The listing builds one solid part. Answer for the finished solid, in the listing's coordinates (mm). Face numbers are marked on the shaded views. Round coordinates to 2 decimals unless told otherwise and drop trailing zeros. Write each loop counter-clockwise with the first axis right and the second up, starting at its lowest first coordinate (ties: lowest second). Pieces come first, ordered by that corner, then holes. Notation, with made-up numbers: (25, -36.75) - (84, -36.75) arc R18 ccw to (84, -17.75) - close; hole circle Ø1 at (-25.5, -13.5). An arc over 180 degrees is marked (long way). Answer as CSV lines item,"result". Start each with the question number.
Item 1: A cutting plane is placed at D-D on x = -5.25. Determine the outline of the cut face in (y, z).
Item 2: A cutting plane is placed at A-A on z = 2.5. Determine the outline of the cut face in (x, y), and give its area (3 significant figures).
Item 3: Flat-ended cylindrical pins translate along their axes: pin 1 (1 mm diameter, centred on x = 4, y = 1, fed in from -Z); pin 2 (1.8 mm diameter, centred on x = -8, z = -2.5, fed in from +Y); pin 3 (0.6 mm diameter, centred on x = 8.5, y = 1.5, fed in from -Z); pin 4 (1 mm diameter, centred on y = 1, z = 0, fed in from +X). Find the tip coordinate at first contact, or state that the pin passes through.
Item 4: For a pull along X with two mould halves and no side action, classify the marked faces 1 and 2 as pulls with the +X half, pulls with the -X half, needs draft (parallel to the pull), parting line crosses it, or undercut.
Item 5: A cutting plane is placed at C-C on x = 8.5. Determine the outline of the cut face in (y, z).
Item 6: A cutting plane is placed at B-B on y = 0.55. Determine the outline of the cut face in (x, z), and give its area (3 significant figures).
Item 7: Straight lines are drawn through the part: line 1 along Z through (x, y) = (8.5, 3.75); line 2 along X through (y, z) = (1.4, -2.5); line 3 along X through (y, z) = (3.75, 2.5). For each, find the intervals that lie inside material, in ascending order. Write a range as [from, to].
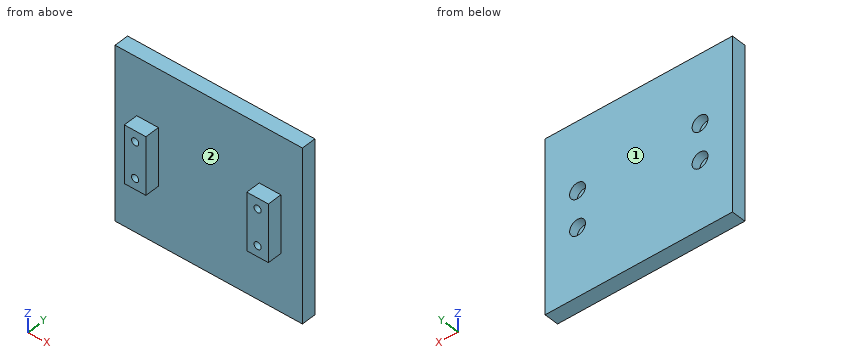
Autodesk Inventor part; units mm, degrees
ref_plane "YZ Plane" through (0, 0, 0) normal (1, 0, 0) x (0, 1, 0)
ref_plane "XZ Plane" through (0, 0, 0) normal (0, 1, 0) x (-1, 0, 0)
ref_plane "XY Plane" through (0, 0, 0) normal (0, 0, 1) x (1, 0, 0)
sketch "Sketch1" plane through (0, 0, 0) normal (0, 0, 1) x (1, 0, 0)
  line L0 (0, 0) -> (10, 0) construction
  line L1 (0, 0) -> (0, 21.2479) construction
  line L2 (10, 0) -> (7, 0)
  line L3 (7, 0) -> (7, 2)
  line L4 (7, 2) -> (0, 2)
  line L5 (10, 0) -> (10, 2)
  line L6 (10, 2) -> (13, 2)
  line L7 (13, 2) -> (13, 4)
  line L8 (13, 4) -> (0, 4)
  line L9 (-7, 0) -> (-7, 2)
  line L10 (-7, 2) -> (0, 2)
  line L11 (-10, 0) -> (-10, 2)
  line L12 (-10, 2) -> (-13, 2)
  line L13 (-13, 2) -> (-13, 4)
  line L14 (-13, 4) -> (0, 4)
  line L15 (-10, 0) -> (-7, 0)
  line L16 (7, 0) -> (10, 0)
  dimension "d0" = 10
  dimension "d1" = 3
  dimension "d2" = 2
  dimension "d3" = 2
  dimension "d4" = 3
  dimension "d5" = 2
extrude "Extrusion1" add sketch "Sketch1" along normal mid plane 8
sketch "Sketch2" plane through (-10, 0, 4) normal (0, -1, 0) x (1, 0, 0)
  line L0 (3, -8) -> (3, 0)
  line L1 (17, -8.5525) -> (20, -8.5525) construction
  line L2 (20, 0.5525) -> (17, 0.5525) construction
  line L3 (0, 0) -> (0, -8) construction
  line L4 (0, -8) -> (3, -8) construction
  line L5 (3, -8) -> (3, 0) construction
  line L6 (3, 0) -> (0, 0) construction
  line L7 (1.5, 0) -> (1.5, -8) construction
  line L8 (18.5, 0.5525) -> (18.5, -8.5525) construction
  line L9 (1.5, -4) -> (18.5, -4) construction
  circle A0 centre (1.5, -1.5) radius 0.5
  line L10 (10, -4) -> (10, 0.5233) construction
  line L11 (18.5, -8.5525) -> (18.5, 0.5525) construction
  circle A1 centre (1.5, -6.5) radius 0.5
  circle A2 centre (18.5, -1.5) radius 0.5
  circle A3 centre (18.5, -6.5) radius 0.5
  line L12 (20, 0) -> (17, 0)
  line L13 (17, -8) -> (17, 0)
  line L14 (17, -8) -> (20, -8)
  line L15 (20, 0) -> (20, -8)
  line L16 (3, -4) -> (17, -4) construction
  line L17 (10, -4) -> (10, -13.0103) construction
  dimension "d8" = 1
  dimension "d9" = 2.5
  dimension "d10" = 0
  dimension "d11" = 0
  dimension "d12" = 8.5
extrude "Extrusion2" cut sketch "Sketch2" against normal through all contours A0 | A1 | A2 | A3
sketch "Sketch3" plane through (-13, 4, 4) normal (0, 1, 0) x (1, 0, 0)
  circle A0 centre (21.5, 6.5) radius 0.5
  circle A1 centre (21.5, 1.5) radius 0.5
  circle A2 centre (4.5, 6.5) radius 0.5
  circle A3 centre (4.5, 1.5) radius 0.5
  circle A4 centre (4.5, 6.5) radius 1.1
  circle A5 centre (4.5, 1.5) radius 1.1
  circle A6 centre (21.5, 6.5) radius 1.1
  circle A7 centre (21.5, 1.5) radius 1.1
  dimension "d15" = 2.2
extrude "Extrusion3" cut sketch "Sketch3" against normal blind 1.2
sketch "Sketch4" plane through (-13, 4, 4) normal (0, 1, 0) x (1, 0, 0)
  line L0 (0, 8) -> (0, 0)
  line L1 (0, 8) -> (26, 8)
  line L2 (26, 8) -> (26, 16)
  line L3 (26, 16) -> (0, 16)
  line L4 (0, 16) -> (0, 8)
  line L5 (0, 0) -> (26, 0)
  line L6 (26, 0) -> (26, -8)
  line L7 (26, -8) -> (0, -8)
  line L8 (0, -8) -> (0, 0)
extrude "Extrusion4" add sketch "Sketch4" against normal up to surface (2 mm away)
properties part number "Table"
Geometry says:
1,outline,"(2, -12) - (4, -12) - (4, 12) - (2, 12) - close"
2,outline,"(-13, 2) - (-10, 2) - (-10, 0) - (-9, 0) - (-9, 2.8) - (-9.6, 2.8) - (-9.6, 4) - (-13, 4) - close; (-8, 0) - (-7, 0) - (-7, 2) - (7, 2) - (7, 0) - (8, 0) - (8, 2.8) - (7.4, 2.8) - (7.4, 4) - (-7.4, 4) - (-7.4, 2.8) - (-8, 2.8) - close; (9, 0) - (10, 0) - (10, 2) - (13, 2) - (13, 4) - (9.6, 4) - (9.6, 2.8) - (9, 2.8) - close"
2,area,"53.1 mm^2"
3,pin 1,"passes through"
3,pin 2,"stops at y = 4"
3,pin 3,"stops at z = -4"
3,pin 4,"stops at x = 10"
4,face 1,"needs draft"
4,face 2,"undercut"
5,outline,"(0, -4) - (2, -4) - (2, -12) - (4, -12) - (4, -3.6) - (2.8, -3.6) - (2.8, -3) - (0, -3) - close; (0, -2) - (2.8, -2) - (2.8, -1.4) - (4, -1.4) - (4, 1.4) - (2.8, 1.4) - (2.8, 2) - (0, 2) - close; (0, 3) - (2.8, 3) - (2.8, 3.6) - (4, 3.6) - (4, 12) - (2, 12) - (2, 4) - (0, 4) - close"
6,outline,"(-10, -4) - (-7, -4) - (-7, 4) - (-10, 4) - close; (7, -4) - (10, -4) - (10, 4) - (7, 4) - close; hole circle Ø1 at (-8.5, -2.5); hole circle Ø1 at (-8.5, 2.5); hole circle Ø1 at (8.5, -2.5); hole circle Ø1 at (8.5, 2.5)"
6,area,"44.9 mm^2"
7,line 1,"z = [-12, -3.6], [-1.4, 1.4], [3.6, 12]"
7,line 2,"x = [-10, -9], [-8, -7], [7, 8], [9, 10]"
7,line 3,"x = [-13, -9.6], [-7.4, 7.4], [9.6, 13]"
